```python
from build123d import *

# Parameters (mm, degrees)
REVOLVE6_ANGLE     = 180
CUT_EXTRUDE3_DEPTH = 34.397155568
SKETCH6_W          = 20.606544016
SKETCH6_H          = 25.002606738
CUT_EXTRUDE4_DEPTH = 3
SKETCH15_W         = 5.12502067
SKETCH15_H         = 26.452748528
CUT_EXTRUDE7_DEPTH = 2
CIRPATTERN1_COUNT  = 6
SKETCH20_R         = 1.6
CUT_EXTRUDE8_DEPTH = 30.260079699


with BuildPart() as part:
    # Sketch1 → Revolve6 (revolve)
    with BuildSketch(Plane.XY):
        with BuildLine():
            Line((0, 24.3), (0, -8.1))
            ThreePointArc((0, -8.1), (16.2, 8.1), (0, 24.3))
        make_face()
    revolve(axis=Axis((0, 24.3, 0), (0, -1, 0)), revolution_arc=REVOLVE6_ANGLE)

    # Sketch7 → Cut-Extrude3 (cut, through all)
    with BuildSketch(Plane(origin=(0, 0, 0), x_dir=(-1, 0, 0), z_dir=(0, 0, -1))):
        with BuildLine():
            Line((-10.303272008, 20.601303369), (10.303272008, 20.601303369))
            ThreePointArc((10.303272008, 20.601303369), (0, 24.3), (-10.303272008, 20.601303369))
        make_face()
        with BuildLine():
            Line((-10.303272008, -4.401303369), (10.303272008, -4.401303369))
            ThreePointArc((10.303272008, -4.401303369), (0, -8.1), (-10.303272008, -4.401303369))
        make_face()
    extrude(amount=-CUT_EXTRUDE3_DEPTH, mode=Mode.SUBTRACT)

    # Sketch6 → Cut-Extrude4 (cut)
    with BuildSketch(Plane(origin=(0, 0, 0), x_dir=(-1, 0, 0), z_dir=(0, 0, -1))):
        with Locations((0, 8.1)):
            Rectangle(SKETCH6_W, SKETCH6_H)
    extrude(amount=-CUT_EXTRUDE4_DEPTH, mode=Mode.SUBTRACT)

    # Sketch15 → Cut-Extrude7 (cut, symmetric)
    with BuildSketch(Plane(origin=(0, 0, 0), x_dir=(0, 0, -1), z_dir=(1, 0, 0))):
        with Locations((-15.573988478, 7.374929105)):
            Rectangle(SKETCH15_W, SKETCH15_H)
    cut_extrude7 = extrude(amount=CUT_EXTRUDE7_DEPTH, both=True, mode=Mode.SUBTRACT)

    # CirPattern1: Cut-Extrude7 ×6 about axis
    cirpattern1_axis = Axis((0, 0, 0), (0, 1, 0))
    for i in range(1, CIRPATTERN1_COUNT):
        add(cut_extrude7.rotate(cirpattern1_axis, i * 360 / CIRPATTERN1_COUNT), mode=Mode.SUBTRACT)

    # Sketch20 → Cut-Extrude8 (cut, through all)
    with BuildSketch(Plane.XY.offset(13.011478143)):
        with Locations((0, 13.267578614)):
            Circle(SKETCH20_R)
        with Locations((0, 4.215406421)):
            Circle(SKETCH20_R)
    extrude(amount=-CUT_EXTRUDE8_DEPTH, mode=Mode.SUBTRACT)


solid = part.part
```
Here's how the part is built. I have some questions about the finished solid (model axes, mm). A direction names the side the tool comes from. Give positions to 0.01 mm unless a question says otherwise; leave off trailing zeros. Loops run counter-clockwise (first coordinate to the right, second up) from the corner with the lowest first, then second, coordinate; pieces in that order, holes last. Notation, with made-up numbers: (80.25, 34.25) -> (101.25, 34.25) arc R11 cw to (101.25, 43.25) -> close; hole circle Ø6 at (20, 47.25). An arc over 180 degrees is marked (long way). Use one line per item in the form item = value. Start each with the question number.
1) Imagine slicing it at D-D (y = 1.5). Please give me the cut outline in (x, z).
2) Imagine slicing it at B-B (y = 12.5). Please give me the cut outline in (x, z), then the cut area to 3 significant figures.
3) Thinking about a two-plate mould opening in X: for faces 6 (the face through (11.319, 8.232, 8.844)), 7 (the face through (-13, 8, 0)), 8 (the face through (10.303, 8, 1)), which applies, +X half, -X half, draft (parallel to the pull), parting line (faces both ways), or undercut?
4) Imagine slicing it at C-C (x = 11.5). Please give me the cut outline in (y, z).
5) Which directions (+Z, -Z, +X, -X, +Y, -Y) give clear straight access to the entire face, cutting with the end or side of a thin tool? Please do faces 1 (the face through (-0.347, 11.706, 8.076)), 2 (the face through (-11.254, 7.965, 6.53)), 3 (the face through (-11.319, 8.232, 8.844)), 4 (the face through (0, 8, 13.011)), 5 (the face through (0, 8, 3)).
6) For P1, Ø3.5, axis at y = 12.5, z = 1, coming from the -X side; P2, Ø3.5, axis at y = 12, z = 14.5, coming from the +X side; P3, Ø3, axis at y = 15.5, z = 4, coming from the +X side; P4, Ø1.5, axis at x = -0.5, z = 10.5, coming from the -Y side, each with a flat end and sliding along its axis, tell me the tip position at first contact or that it passes through.
7) Please list where these lines run through material, in increasing order: line 1 along Y through (x, z) = (0, 8.5); line 2 along X through (y, z) = (10, 2.5); line 3 along Y through (x, z) = (0.5, 5.25).
8) Imagine slicing it at A-A (x = 0). Please give me the cut outline in (y, z).
Check values:
q1.outline = (-14.79, 0) -> (-10.3, 0) -> (-10.3, 3) -> (10.3, 3) -> (10.3, 0) -> (14.79, 0) arc R14.79 ccw to (13.69, 5.6) -> (12.27, 4.77) -> (10.27, 8.24) -> (11.69, 9.06) arc R14.79 ccw to (2, 14.66) -> (2, 13.01) -> (-2, 13.01) -> (-2, 14.66) arc R14.79 ccw to (-11.69, 9.06) -> (-10.27, 8.24) -> (-12.27, 4.77) -> (-13.69, 5.6) arc R14.79 ccw to start
q2.outline = (-15.59, 0) -> (-10.3, 0) -> (-10.3, 3) -> (-1.4, 3) -> (-1.4, 13.01) -> (-2, 13.01) -> (-2, 15.46) arc R15.59 ccw to (-12.39, 9.46) -> (-10.27, 8.24) -> (-12.27, 4.77) -> (-14.39, 6) arc R15.59 ccw to start; (1.4, 3) -> (10.3, 3) -> (10.3, 0) -> (15.59, 0) arc R15.59 ccw to (14.39, 6) -> (12.27, 4.77) -> (10.27, 8.24) -> (12.39, 9.46) arc R15.59 ccw to (2, 15.46) -> (2, 13.01) -> (1.4, 13.01) -> close
q2.area = 261 mm^2
q3.face_6 = +X half
q3.face_7 = draft
q3.face_8 = undercut
q4.outline = (-3.31, 0) -> (19.51, 0) arc R11.41 ccw to (17.74, 6.1) -> (-1.54, 6.1) arc R11.41 ccw to start; (1.02, 8.95) -> (15.18, 8.95) arc R11.41 ccw to start
q5.face_1 = +Z, -Z
q5.face_2 = +Y, -Y
q5.face_3 = -X, +Y, -Y
q5.face_4 = +Z, +Y, -Y
q5.face_5 = -Z, +Y, -Y
q6.P1 = -15.96
q6.P2 = 9.3
q6.P3 = 14.65
q6.P4 = -4.4
q7.line_1 = -4.4 to 2.62, 5.82 to 11.67, 14.87 to 20.6
q7.line_2 = -15.89 to -10.3, 10.3 to 15.89
q7.line_3 = -4.4 to 2.7, 5.74 to 11.75, 14.79 to 20.6
q8.outline = (-4.4, 3) -> (2.62, 3) -> (2.62, 13.01) -> (-1.55, 13.01) arc R16.2 ccw to (-4.4, 10.3) -> close; (5.82, 3) -> (11.67, 3) -> (11.67, 13.01) -> (5.82, 13.01) -> close; (14.87, 3) -> (20.6, 3) -> (20.6, 10.3) arc R16.2 ccw to (17.75, 13.01) -> (14.87, 13.01) -> close
